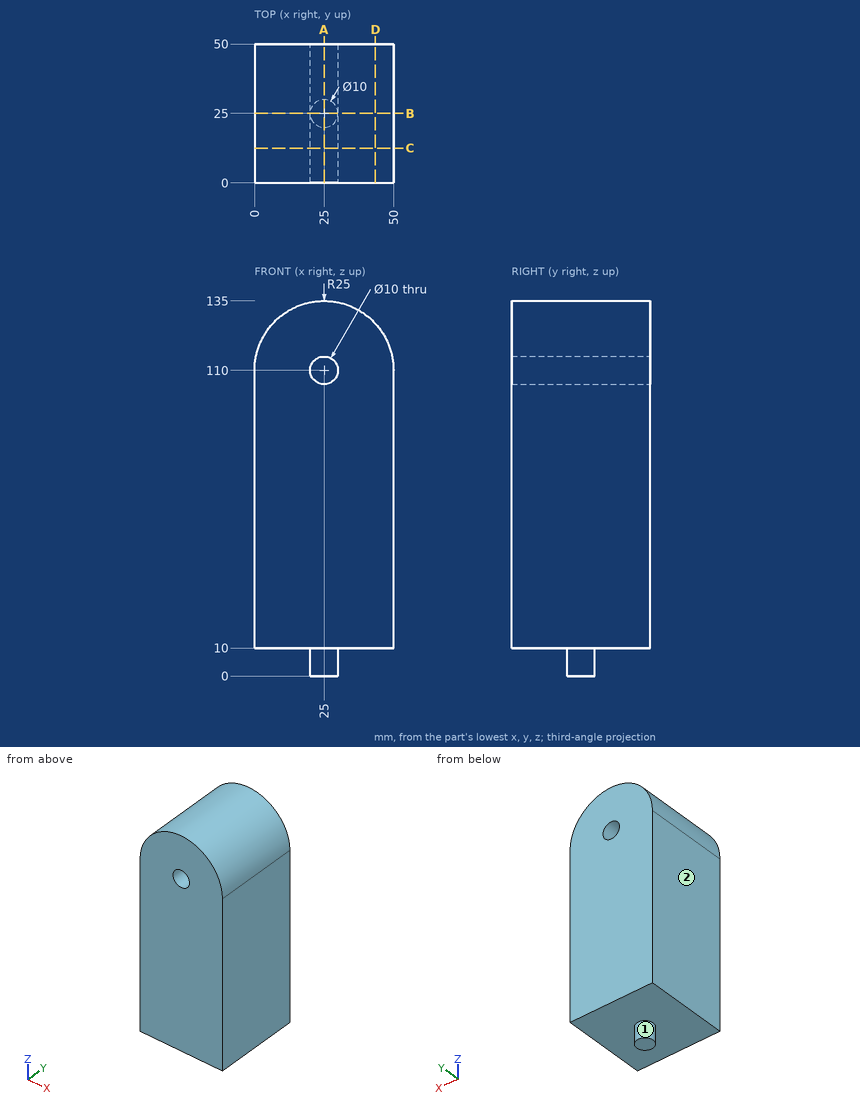
Geometry check sheet. Reference: drawing and pictorial views, mm from the part's lowest x, y, z. A direction names the side the tool comes from. Give positions to 0.01 mm unless a question says otherwise; leave off trailing zeros. Order: outer loops, then holes, each group sorted by start corner. A loop starts at its lowest first (then second) coordinate and runs counter-clockwise, first axis right, second up. Notation, with made-up numbers: M 22.25,34 L 56.25,34 A32 cw 56.25,70 Z; hole C -17,-18.5 d4. An arc over 180 degrees is marked long. Answer as a JSON object with one key per item and string values. Group by question number.
1) Scan lines: line 1 along Z through (x, y) = (25, 19); line 2 along X through (y, z) = (36, 110); line 3 along Z through (x, y) = (21, 35). Record each from-to range of solid material in increasing order. Write a range as [from, to].
2) Cross-section at B-B (y = 25). Enter the section's corners in (x, z).
3) Cross-section at A-A (x = 25). Enter the section's corners in (y, z).
4) Depth check by flat-ended pin: pin 1 Ø10 at (x, y) = (7.5, 8.5) entering from -Z; pin 2 Ø4 at (x, y) = (42.5, 11) entering from +Z; pin 3 Ø6 at (x, y) = (38.5, 39.5) entering from +Z. Enter the tip coordinate at first touch or a pass-through.
5) Cross-section at C-C (y = 12.5). Enter the section's corners in (x, z).
6) Cross-section at D-D (x = 43.5). Enter the section's corners in (y, z).
7) Access from +Z, -Z, +X, -X, +Y, -Y to the whole of each face (thin tool, end or side, straight path). Record for the marked faces 1 and 2.
Result sheet:
{
 "1": {"line 1": "z = [10, 105], [115, 135]", "line 2": "x = [0, 20], [30, 50]", "line 3": "z = [10, 107], [113, 134.68]"},
 "2": {"outline": "M 0,10 L 20,10 L 20,0 L 30,0 L 30,10 L 50,10 L 50,110 A25 ccw 0,110 Z; hole C 25,110 d10"},
 "3": {"outline": "M 0,10 L 20,10 L 20,0 L 30,0 L 30,10 L 50,10 L 50,105 L 0,105 Z; M 0,115 L 50,115 L 50,135 L 0,135 Z"},
 "4": {"pin 1": "stops at z = 10", "pin 2": "stops at z = 129.62", "pin 3": "stops at z = 132.69"},
 "5": {"outline": "M 0,10 L 50,10 L 50,110 A25 ccw 0,110 Z; hole C 25,110 d10"},
 "6": {"outline": "M 0,10 L 50,10 L 50,126.82 L 0,126.82 Z"},
 "7": {"face 1": "-Z", "face 2": "+Z, -Z, -X, +Y, -Y"}
}
